Geometry: see drawing. Coordinates: mm, zero at the bounding-box minimum. A direction names the side the tool comes from. Give positions to 0.01 mm unless a question says otherwise; leave off trailing zeros. Loops run counter-clockwise (first coordinate to the right, second up) from the corner with the lowest first, then second, coordinate; pieces in that order, holes last. Notation, with made-up numbers: M 10.5,-6 L 17.5,-6 A11 ccw 17.5,3 Z; hole C 19,70 d1. An arc over 180 degrees is marked long. Return JSON: item names as keys, results as strings. Group by question number.
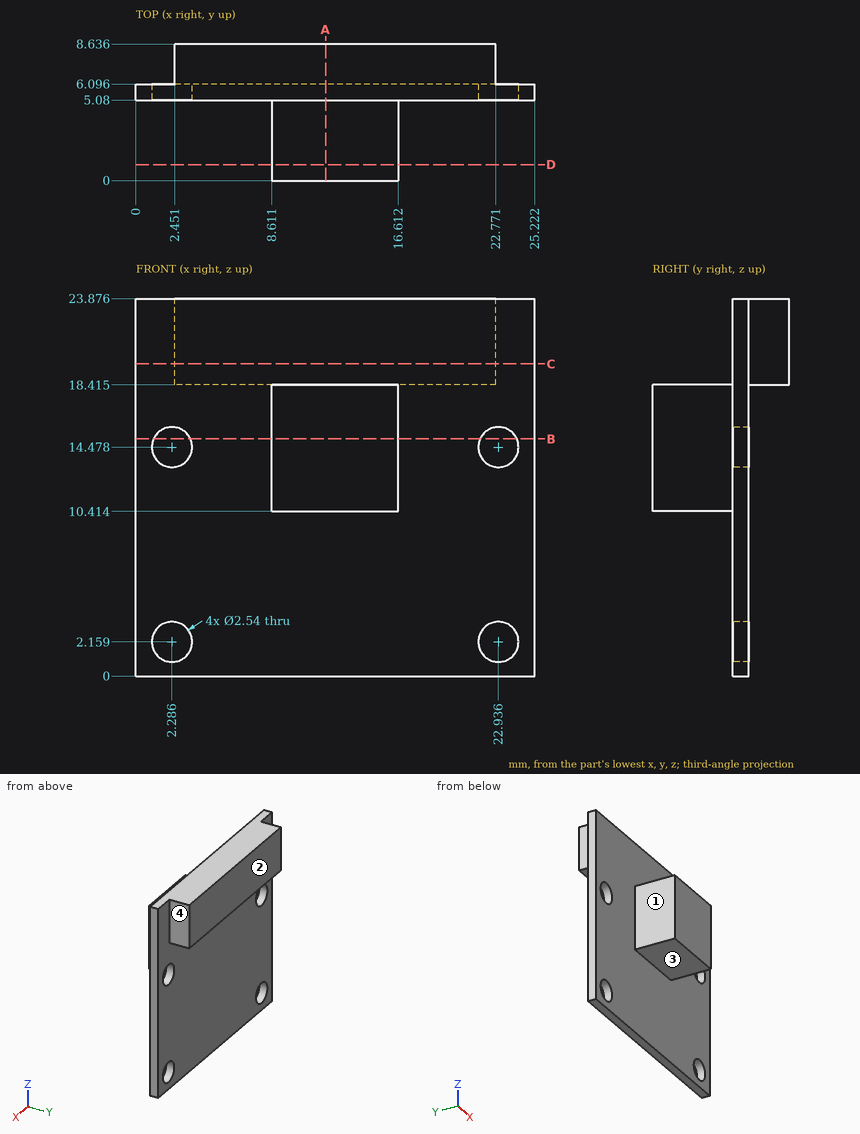
Item 1: Section C-C, the plane z = 19.75. Return loops of the section in (x, y).
Item 2: Section A-A, the plane x = 12. Return loops of the section in (y, z) (1 decimal).
Item 3: Material intervals for line 1 (X direction, y = 4.75, z = 16); line 2 (Y direction, x = 14, z = 5); line 3 (Z direction, x = 6, y = 7) (1 decimal), sorted ascending. Write a range as from..to.
Item 4: First-contact query: pin 1 Ø1 at (y, z) = (4.5, 4.5) entering from +X; pin 2 Ø1 at (y, z) = (3.5, 17) entering from +X; pin 3 Ø3 at (x, z) = (22.94, 14.48) entering from -Y; pin 4 Ø0.8 at (x, y) = (14, 7.5) entering from -Z (3 decimals). Flat tips, straight axial feed; report the tip coordinate or a pass-through.
Item 5: Reachability of the marked faces 1, 2, 3 and 4 from +Z, -Z, +X, -X, +Y, -Y: full face, straight path, thin tool, end or side. Return the list, or none.
Item 6: Section D-D, the plane y = 1. Return loops of the section in (x, z) (1 decimal), then the cut area to 3 significant figures.
Item 7: Section B-B, the plane z = 15. Return loops of the section in (x, y).
Answer below:
{
 "1": {"outline": "M 0,5.08 L 25.22,5.08 L 25.22,6.1 L 22.77,6.1 L 22.77,8.64 L 2.45,8.64 L 2.45,6.1 L 0,6.1 Z"},
 "2": {"outline": "M 0,10.4 L 5.1,10.4 L 5.1,0 L 6.1,0 L 6.1,18.4 L 8.6,18.4 L 8.6,23.9 L 5.1,23.9 L 5.1,18.4 L 0,18.4 Z"},
 "3": {"line 1": "8.61..16.61", "line 2": "5.08..6.1", "line 3": "18.4..23.9"},
 "4": {"pin 1": "through", "pin 2": "x = 16.61", "pin 3": "y = 5.08", "pin 4": "z = 18.415"},
 "5": {"face 1": "+Z, -Z, -X, -Y", "face 2": "+Z, -Z, +X, -X, +Y", "face 3": "-Z, +X, -X, -Y", "face 4": "+Z, -Z, +X, +Y"},
 "6": {"outline": "M 8.6,10.4 L 16.6,10.4 L 16.6,18.4 L 8.6,18.4 Z", "area": "64.0 mm^2"},
 "7": {"outline": "M 0,5.08 L 1.13,5.08 L 1.13,6.1 L 0,6.1 Z; M 3.44,5.08 L 8.61,5.08 L 8.61,0 L 16.61,0 L 16.61,5.08 L 21.78,5.08 L 21.78,6.1 L 3.44,6.1 Z; M 24.09,5.08 L 25.22,5.08 L 25.22,6.1 L 24.09,6.1 Z"}
}
